Solid Edge part; units mm, degrees
sketch "Sketch1" plane through (0, 0, 0) normal (0, -1, 0) x (1, 0, 0)
  line L0 (-13.5, 13) -> (-13.5, 0)
  line L1 (-13.5, 0) -> (13.5, 0)
  line L2 (13.5, 0) -> (13.5, 13)
  line L3 (13.5, 13) -> (33.5, 13)
  line L4 (33.5, 13) -> (33.5, 11)
  line L5 (33.5, 11) -> (15.5, 11)
  line L6 (15.5, 11) -> (15.5, -2)
  line L7 (15.5, -2) -> (-15.5, -2)
  line L8 (-15.5, -2) -> (-15.5, 11)
  line L9 (-15.5, 11) -> (-35.5, 11)
  line L10 (-35.5, 11) -> (-35.5, 13)
  line L11 (-35.5, 13) -> (-13.5, 13)
extrude "Protrusion1" add sketch "Sketch1" against normal blind 20
sketch "Sketch2" plane through (-1, 0, 5.5) normal (0, -1, 0) x (1, 0, 0)
  line L0 (21.5, 5.5) -> (21.5, -7.5)
  line L1 (21.5, -7.5) -> (-14.5, -7.5)
  line L2 (-14.5, -7.5) -> (-14.5, 5.5)
  line L3 (-14.5, 5.5) -> (-34.5, 5.5)
  line L4 (-34.5, 5.5) -> (-34.5, 7.5)
  line L5 (-34.5, 7.5) -> (-12.5, 7.5)
  line L6 (-12.5, 7.5) -> (-12.5, -5.5)
  line L7 (-12.5, -5.5) -> (19.5, -5.5)
  line L8 (19.5, -5.5) -> (19.5, 7.5)
  line L9 (19.5, 7.5) -> (39.5, 7.5)
  line L10 (39.5, 7.5) -> (39.5, 5.5)
  line L11 (39.5, 5.5) -> (21.5, 5.5)
extrude "ExtrudedProtrusion_2" add sketch "Sketch2" against normal blind 30
sketch "Sketch3" plane through (26, 15, 13) normal (0, 0, 1) x (1, 0, 0)
  line L0 (-12.5, -15) -> (-12.5, 5)
  line L1 (-12.5, 5) -> (-7.5, 5)
  line L2 (-7.5, 5) -> (-7.5, -15)
  line L3 (-7.5, -15) -> (-12.5, -15)
extrude "Cutout1" cut sketch "Sketch3" against normal up to next
sketch "Sketch4" plane through (2.5, 15, -2) normal (0, 0, -1) x (1, 0, 0)
  line L0 (11, -5) -> (16, -5)
  line L1 (16, -5) -> (16, 15)
  line L2 (16, 15) -> (10.9467, 15)
  line L3 (10.9467, 15) -> (11, -5)
extrude "ExtrudedProtrusion_3" add sketch "Sketch4" against normal blind 2
sketch "Sketch5" plane through (-24.5, 15, 13) normal (0, 0, 1) x (0, 1, 0)
  line L0 (15, -6) -> (-15, -6)
  line L1 (-15, -6) -> (-15, 11)
  line L2 (-15, 11) -> (15, 11)
  line L3 (15, 11) -> (15, -6)
  line L4 (-15, -48) -> (15, -48)
  line L5 (15, -48) -> (15, -63)
  line L6 (15, -63) -> (-15, -63)
  line L7 (-15, -63) -> (-15, -48)
extrude "Cutout2" cut sketch "Sketch5" against normal up to next
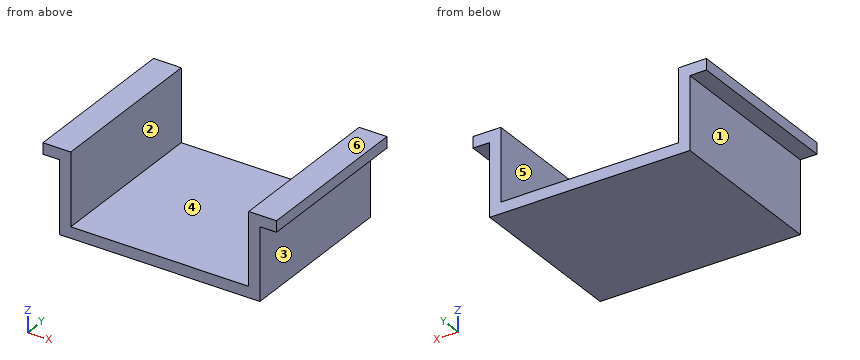
CAD build for the part. Positions are in the model's coordinates, mm. Face numbers are marked on the shaded views. A direction names the side the tool comes from. Coordinates: 2 decimals unless noted, no trailing zeros. Order: outer loops, then holes, each group sorted by start corner. A loop starts at its lowest first (then second) coordinate and runs counter-clockwise, first axis right, second up. Notation, with made-up numbers: M 72.25,-12 L 130.25,-12 A23 cw 130.25,-2 Z; hole C -3.75,75 d8. An arc over 180 degrees is marked long. Write each question's results on one line, items separated by ' | '. Start each with the question number.
Q1. Cut at A-A (z = 8.75). List the corners of the cut face in (x, y), then the cut area to 3 significant figures.
Q2. Which spindle directions (+Z, -Z, +X, -X, +Y, -Y) get a long thin tool onto all of the face, cutting with end or side? Do the marked faces 5 and 6. Say none if no direction does.
Q3. Cut at C-C (x = -9). List the corners of the cut face in (y, z), then the cut area to 3 significant figures.
Q4. Flat gauge pins, fed straight in: P1, Ø2, axis at x = -8.5, z = 1.5, coming from the -Y side; P2, Ø4, axis at x = 3, y = 14.5, coming from the +Z side; P3, Ø8, axis at y = 24, z = 0.5, coming from the -X side; P4, Ø2, axis at y = 14.5, z = 7, coming from the +X side. Where does each tip first touch, or does it go through?
Q5. Pull direction X, two halves, no side cores. Call the marked faces 1, 2, 3 and 4: +X half, -X half, draft (parallel to the pull), parting line (faces both ways), or undercut.
Q6. Cut at B-B (y = 11.75). List the corners of the cut face in (x, z).
Q7. Cut at D-D (z = -1). List the corners of the cut face in (x, y), then the cut area to 3 significant figures.
Q8. Drill centre lines: probe 1 along X at (y, z) = (12.5, 9.75); probe 2 along Z at (x, y) = (-0.5, 20.25); probe 3 along Z at (x, y) = (21, 25.5). Where is each one in solid material? Low to high. Write a range as from..to.
Found:
1) outline: M -15.5,0 L -13.5,0 L -13.5,30 L -15.5,30 Z; M 18.5,0 L 20.5,0 L 20.5,30 L 18.5,30 Z | area: 120 mm²
2) face 5: +Z, +Y, -Y | face 6: +Z, +X, -X, +Y, -Y
3) outline: M 0,-2 L 30,-2 L 30,0 L 0,0 Z | area: 60.0 mm²
4) P1: through | P2: z = 0 | P3: x = -15.5 | P4: x = 20.5
5) face 1: -X half | face 2: undercut | face 3: +X half | face 4: undercut
6) outline: M -18.5,11 L -15.5,11 L -15.5,-2 L 20.5,-2 L 20.5,11 L 23.5,11 L 23.5,13 L 18.5,13 L 18.5,0 L -13.5,0 L -13.5,13 L -18.5,13 Z
7) outline: M -15.5,0 L 20.5,0 L 20.5,30 L -15.5,30 Z | area: 1,080 mm²
8) probe 1: -15.5..-13.5, 18.5..20.5 | probe 2: -2..0 | probe 3: 11..13
